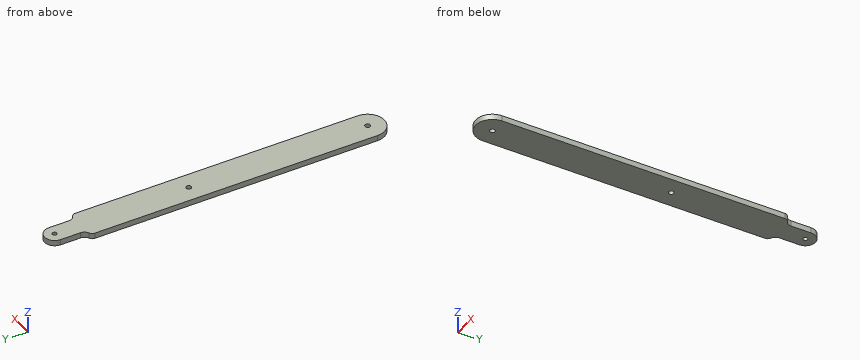
from build123d import *

# Parameters (mm, degrees)
SKETCH1_R           = 1.4605
SKETCH1_R_2         = 1.27
BOSS_EXTRUDE1_DEPTH = 3.175
SKETCH3_R           = 1.4605
CUT_EXTRUDE2_DEPTH  = 3.175


with BuildPart() as part:
    # Sketch1 → Boss-Extrude1 (new body)
    with BuildSketch(Plane.XY):
        with BuildLine():
            Line((-19.353012887, 135.150128867), (-19.353012887, -25.400000121))
            ThreePointArc((-19.353012887, -25.400000121), (-9.828012887, -34.925000121), (-0.303012887, -25.400000121))
            Line((-0.303012887, -25.400000121), (-0.303012887, 135.150128867))
            ThreePointArc((-0.303012887, 135.150128867), (-0.71789642, 136.541344163), (-1.827012887, 137.47807732))
            ThreePointArc((-1.827012887, 137.47807732), (-3.490687589, 138.883177056), (-4.113012887, 140.97))
            Line((-4.113012887, 140.97), (-4.113012887, 152.4))
            ThreePointArc((-4.113012887, 152.4), (-9.828012887, 158.115), (-15.543012887, 152.4))
            Line((-15.543012887, 152.4), (-15.543012887, 140.97))
            ThreePointArc((-15.543012887, 140.97), (-16.165338186, 138.883177056), (-17.829012887, 137.47807732))
            ThreePointArc((-17.829012887, 137.47807732), (-18.938129355, 136.541344163), (-19.353012887, 135.150128867))
        make_face()
        with Locations((-9.828012887, -25.400000121)):
            Circle(SKETCH1_R, mode=Mode.SUBTRACT)
        with Locations((-9.828012887, 152.4)):
            Circle(SKETCH1_R_2, mode=Mode.SUBTRACT)
    extrude(amount=BOSS_EXTRUDE1_DEPTH)

    # Sketch3 → Cut-Extrude2 (cut)
    with BuildSketch(Plane.XY.offset(3.175)):
        with Locations((-9.828012887, 76.2)):
            Circle(SKETCH3_R)
    extrude(amount=-CUT_EXTRUDE2_DEPTH, mode=Mode.SUBTRACT)


solid = part.part
Work out the finished part from the listing and answer in its coordinate system (mm). Coordinates: 2 decimals unless noted, no trailing zeros.
1. A flat-ended cylindrical pin translates along its axis: pin 1 (1.6 mm diameter, centred on y = 148, z = 2, fed in from -X). Find the tip coordinate at first contact, or state that the pin passes through.
Results list:
pin 1: stops at x = -15.54
2. The part is cut by section A-A, the plane z = 0.85. State how many separate pieces and enclosed holes the cut face has, and give its area (3 significant figures).
Results list:
separate pieces: 1
enclosed holes: 3
area: 3,450 mm2
3. Consider line 1 along Y through (x, z) = (-9.75, 2.65); line 2 along X through (y, z) = (76.2, 1.3); line 3 along Y through (x, z) = (-8.5, 0.4). Determine where each line is inside the solid, lowest interval first.
Results list:
line 1: y = -34.92 to -26.86, -23.94 to 74.74, 77.66 to 151.13, 153.67 to 158.11
line 2: x = -19.35 to -11.29, -8.37 to -0.3
line 3: y = -34.83 to -26.01, -24.79 to 75.59, 76.81 to 157.96
